Verification items for the finished model (mm, model axes). A direction names the side the tool comes from. Coordinates: 2 decimals unless noted, no trailing zeros. Order: outer loops, then holes, each group sorted by start corner. A loop starts at its lowest first (then second) coordinate and runs counter-clockwise, first axis right, second up. Notation, with made-up numbers: M 86,0.25 L 108,0.25 A16 ccw 108,6.25 Z; hole C 29,61 d7. An arc over 180 degrees is marked long. Return JSON: item names as keys, results as strings.
```python
from build123d import *

# Parameters (mm, degrees)
SKETCH1_W                 = 45
SKETCH1_H                 = 15
BOSS_EXTRUDE1_DEPTH       = 60
SHELL1_T                  = -4
SHELL1_THICKNESS_2_FACE_W = 7
SHELL1_THICKNESS_2_FACE_H = 37
SHELL1_THICKNESS_2_DEPTH  = 2
SKETCH3_W                 = 10
SKETCH3_H                 = 7
CUT_EXTRUDE2_DEPTH        = 4
CUT_EXTRUDE3_REACH        = 67.812
SKETCH4_W                 = 10
SKETCH4_H                 = 10
SKETCH5_W                 = 7.4
SKETCH5_H                 = 7.4
CUT_EXTRUDE4_DEPTH        = 76.374067158
CUT_EXTRUDE5_START        = -1.2
CUT_EXTRUDE5_DEPTH        = 3.6
CUT_EXTRUDE6_REACH        = 124.321
SKETCH7_R                 = 2.1


with BuildPart() as part:
    # Sketch1 → Boss-Extrude1 (new, symmetric)
    with BuildSketch(Plane(origin=(0, 0, 0), x_dir=(1, 0, 0), z_dir=(0, 1, 0))):
        Rectangle(SKETCH1_W, SKETCH1_H)
    extrude(amount=BOSS_EXTRUDE1_DEPTH, both=True)

    # Shell1
    shell1_openings = [part.faces().sort_by_distance(p)[0] for p in [
        (0, 60, 0),
    ]]
    offset(amount=SHELL1_T, openings=shell1_openings, kind=Kind.INTERSECTION)

    # Shell1 thickness 2 face (on inner face of the shell) → Shell1 thickness 2 (add)
    with BuildSketch(Plane(origin=(0, -56, 0), x_dir=(0, 0, -1), z_dir=(0, -1, 0))):
        Rectangle(SHELL1_THICKNESS_2_FACE_W, SHELL1_THICKNESS_2_FACE_H)
    extrude(amount=-SHELL1_THICKNESS_2_DEPTH)

    # Sketch3 → Cut-Extrude2 (cut)
    with BuildSketch(Plane.XZ.offset(60)):
        Rectangle(SKETCH3_W, SKETCH3_H)
    extrude(amount=-CUT_EXTRUDE2_DEPTH, mode=Mode.SUBTRACT)

    # Sketch4 → Cut-Extrude3 (cut, up to next)
    with BuildSketch(Plane.XY.offset(7.5), mode=Mode.PRIVATE) as cut_extrude3_sk1:
        with Locations((0, 45)):
            Rectangle(SKETCH4_W, SKETCH4_H)
    cut_extrude3_tool1 = extrude(cut_extrude3_sk1.sketch, amount=-CUT_EXTRUDE3_REACH, mode=Mode.PRIVATE) & part.part
    add(cut_extrude3_tool1.solids().sort_by_distance((0, 45, 7.5))[0], mode=Mode.SUBTRACT)

    # Sketch5 → Cut-Extrude4 (cut, through all)
    with BuildSketch(Plane(origin=(22.5, 0, 0), x_dir=(0, 0, -1), z_dir=(1, 0, 0))):
        with Locations((0, 43.5)):
            Rectangle(SKETCH5_W, SKETCH5_H)
    extrude(amount=-CUT_EXTRUDE4_DEPTH, mode=Mode.SUBTRACT)

    # Sketch6 → Cut-Extrude5 (cut)
    with BuildSketch(Plane.XZ.offset(60).offset(CUT_EXTRUDE5_START)):
        Polygon((-15, 4.272391992), (-18.7, 2.136195996), (-18.7, -2.136195996), (-15, -4.272391992), (-11.3, -2.136195996), (-11.3, 2.136195996), align=None)
        Polygon((11.3, 2.136195996), (15, 4.272391992), (18.7, 2.136195996), (18.7, -2.136195996), (15, -4.272391992), (11.3, -2.136195996), align=None)
    extrude(amount=-CUT_EXTRUDE5_DEPTH, mode=Mode.SUBTRACT)

    # Sketch7 → Cut-Extrude6 (cut, up to next)
    with BuildSketch(Plane.XZ.offset(60), mode=Mode.PRIVATE) as cut_extrude6_sk1:
        with Locations(Location((-15, 0, 0), (0, 0, 270))):
            Circle(SKETCH7_R)
    cut_extrude6_tool1 = extrude(cut_extrude6_sk1.sketch, amount=-CUT_EXTRUDE6_REACH, mode=Mode.PRIVATE) & part.part
    # Sketch7 → Cut-Extrude6 (cut, up to next)
    with BuildSketch(Plane.XZ.offset(60), mode=Mode.PRIVATE) as cut_extrude6_sk2:
        with Locations(Location((15, 0, 0), (0, 0, 90))):
            Circle(SKETCH7_R)
    cut_extrude6_tool2 = extrude(cut_extrude6_sk2.sketch, amount=-CUT_EXTRUDE6_REACH, mode=Mode.PRIVATE) & part.part
    add(cut_extrude6_tool1.solids().sort_by_distance((-15, -60, 0))[0], mode=Mode.SUBTRACT)
    add(cut_extrude6_tool2.solids().sort_by_distance((15, -60, 0))[0], mode=Mode.SUBTRACT)


solid = part.part
```
Q1. Go/stop test with a flat-tipped pin: pin 1 (4 mm diameter, centred on x = 15, z = 0, fed in from +Y). Record where the tip stops, or that it passes through.
Values:
{"pin 1": "y = -54"}
Q2. Cross-section at C-C, the plane y = -3. Record the boundary of the cut face in (x, z), and give its area (3 significant figures).
Values:
{"outline": "M -22.5,-7.5 L 22.5,-7.5 L 22.5,7.5 L -22.5,7.5 Z; hole M -18.5,-3.5 L 18.5,-3.5 L 18.5,3.5 L -18.5,3.5 Z", "area": "416 mm^2"}
Q3. Tool access check on faces 1 (the face through (16.876, -57.025, -3.189)), 2 (the face through (-5, -58, 0)), 3 (the face through (5.3, 43.4, 3.7)), 4 (the face through (-5, 45, 6)), 5 (the face through (0, -6, -3.5)). Record the directions out of +Z, -Z, +X, -X, +Y, -Y that give a thin tool (end or side, any length) a straight path to the whole face; none if there is none.
Values:
{"face 1": "none", "face 2": "-Y", "face 3": "+X, -X", "face 4": "+Z", "face 5": "+Y"}
Q4. Cross-section at A-A, the plane x = 2. Record the boundary of the cut face in (y, z).
Values:
{"outline": "M -60,-7.5 L 60,-7.5 L 60,-3.5 L 47.2,-3.5 L 47.2,-3.7 L 39.8,-3.7 L 39.8,-3.5 L -54,-3.5 L -54,3.5 L 39.8,3.5 L 39.8,3.7 L 40,3.7 L 40,7.5 L -60,7.5 L -60,3.5 L -56,3.5 L -56,-3.5 L -60,-3.5 Z; M 50,3.5 L 60,3.5 L 60,7.5 L 50,7.5 Z"}
Q5. Draft check along X on faces 6 (the face through (0, 1, 7.5)), 7 (the face through (18.5, 54, 0)). Enter one of: pulls with the +X half, pulls with the -X half, needs draft (parallel to the pull), parting line crosses it, or undercut.
Values:
{"face 6": "needs draft", "face 7": "undercut"}
Q6. Cross-section at B-B, the plane y = 42.5. Record the boundary of the cut face in (x, z).
Values:
{"outline": "M -22.5,-7.5 L 22.5,-7.5 L 22.5,-3.7 L -22.5,-3.7 Z; M -22.5,3.7 L -5,3.7 L -5,7.5 L -22.5,7.5 Z; M 5,3.7 L 22.5,3.7 L 22.5,7.5 L 5,7.5 Z"}
Q7. Cross-section at D-D, the plane x = -9. Record the boundary of the cut face in (y, z), and give its area (3 significant figures).
Values:
{"outline": "M -60,-7.5 L 60,-7.5 L 60,-3.5 L 47.2,-3.5 L 47.2,-3.7 L 39.8,-3.7 L 39.8,-3.5 L -54,-3.5 L -54,3.5 L 39.8,3.5 L 39.8,3.7 L 47.2,3.7 L 47.2,3.5 L 60,3.5 L 60,7.5 L -60,7.5 Z", "area": "999 mm^2"}
Q8. Material ranges on line 1 along X through (y, z) = (-59.2, 0); line 2 along Z through (x, y) = (4, -34); line 3 along X through (y, z) = (-27.5, -1.25), recorded low to high.
Values:
{"line 1": "-22.5 to -17.1, -12.9 to -5, 5 to 12.9, 17.1 to 22.5", "line 2": "-7.5 to -3.5, 3.5 to 7.5", "line 3": "-22.5 to -18.5, 18.5 to 22.5"}
